Here's how the part is built. I have some questions about the finished solid (model axes, mm). Face numbers are marked on the shaded views. Round coordinates to 2 decimals unless told otherwise and drop trailing zeros. Loops run counter-clockwise (first coordinate to the right, second up) from the corner with the lowest first, then second, coordinate; pieces in that order, holes last. Notation, with made-up numbers: M -20,-7.5 L 5,-7.5 A9 ccw 5,-3.5 Z; hole C 31.5,84 d8. An arc over 180 degrees is marked long. One line per question, with ' | ' between items. Start each with the question number.
Autodesk Inventor part; units mm, degrees
ref_plane "YZ Plane" through (0, 0, 0) normal (1, 0, 0) x (0, 1, 0)
ref_plane "XZ Plane" through (0, 0, 0) normal (0, 1, 0) x (-1, 0, 0)
ref_plane "XY Plane" through (0, 0, 0) normal (0, 0, 1) x (1, 0, 0)
sketch "Skizze1" plane through (0, 0, 0) normal (0, 0, 1) x (1, 0, 0)
  line L0 (0, 0) -> (32, 0)
  line L1 (32, 0) -> (32, 59)
  line L2 (32, 59) -> (0, 59)
  line L3 (0, 59) -> (0, 0)
  dimension "d0" = 32
  dimension "d1" = 59
extrude "Extrusion1" add sketch "Skizze1" against normal blind 2
sketch "Skizze2" plane through (0, 0, -2) normal (0, 0, -1) x (-1, 0, 0)
  line L0 (-2.1, 2.1) -> (-29.9, 2.1)
  line L1 (-29.9, 2.1) -> (-29.9, 56.9)
  line L2 (-29.9, 56.9) -> (-2.1, 56.9)
  line L3 (-2.1, 56.9) -> (-2.1, 2.1)
  line L4 (0, 0) -> (0, 59) construction
  line L5 (-32, 0) -> (0, 0) construction
  point P0 (-2.1, 29.5)
  point P1 (0, 29.5)
  point P2 (-16, 2.1)
  point P3 (-16, 0)
  dimension "d4" = 2.1
  dimension "d5" = 2.1
extrude "Extrusion2" add sketch "Skizze2" along normal blind 2
sketch "Skizze3" plane through (0, 0, -4) normal (0, 0, -1) x (-1, 0, 0)
  circle A0 centre (-19.7, 39.4) radius 2.7
  line L0 (-32, 0) -> (0, 0)
  line L1 (-2.1, 2.1) -> (-2.1, 56.9)
  line L2 (-29.9, 56.9) -> (-29.9, 2.1)
  circle A1 centre (-19.7, 47.02) radius 2.7
  dimension "d8" = 5.4
  dimension "d9" = 39.4
  dimension "d11" = 10.2
  dimension "d12" = 5.4
  dimension "d13" = 7.62
extrude "Extrusion3" cut sketch "Skizze3" against normal through all
fillet "Rundung1" radius 1 4 edges at (16, 56.9, -4) (29.9, 29.5, -4) (2.1, 29.5, -4) (16, 2.1, -4)
fillet "Rundung2" radius 2 4 edges at (0, 59, -1) (0, 0, -1) (32, 59, -1) (32, 0, -1)
sketch "Skizze4" plane through (0, 0, -4) normal (0, 0, -1) x (-1, 0, 0)
  line L0 (-26, 31.9) -> (-6, 31.9)
  line L1 (-6, 31.9) -> (-6, 35.4)
  line L2 (-6, 35.4) -> (-26, 35.4)
  line L3 (-26, 35.4) -> (-26, 31.9)
  line L4 (-29.9, 2.1) -> (-2.1, 2.1)
  point P0 (0, 0)
  point P1 (-16, 31.9)
  point P2 (-16, 2.1)
  dimension "d18" = 20
  dimension "d19" = 3.5
  dimension "d20" = 29.8
extrude "Extrusion4" add sketch "Skizze4" along normal blind 6.01
sketch "Skizze6" plane through (6, 31.9, -4) normal (0, -1, 0) x (1, 0, 0)
  line L0 (0, -6.01) -> (2.5, -6.01)
  line L1 (2.5, -6.01) -> (0, -2)
  line L2 (0, -2) -> (0, -6.01)
  line L3 (20, 0) -> (0, 0) construction
  line L4 (10, 0) -> (10, 6.9424) construction
  line L5 (20, -6.01) -> (17.5, -6.01)
  line L6 (17.5, -6.01) -> (20, -2)
  line L7 (20, -2) -> (20, -6.01)
  point P0 (-6, 4)
  dimension "d29" = 2
  dimension "d30" = 2.5
  dimension "d31" = 4.01
extrude "Extrusion5" cut sketch "Skizze6" against normal up to surface (3.5 mm away)
properties part number "top"
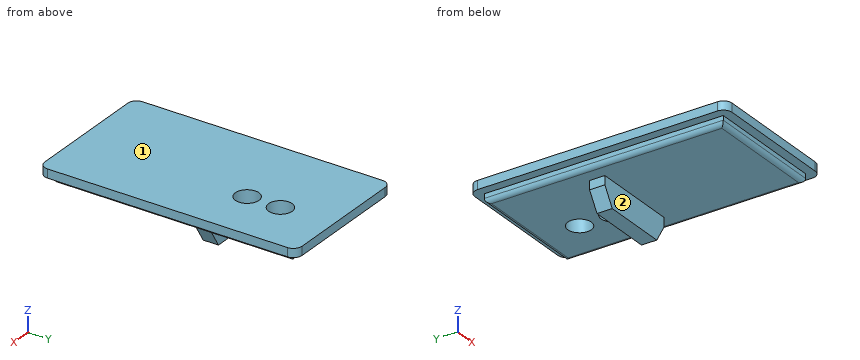
1) Imagine slicing it at B-B (x = 19.7). Write out the boundary of the cut face in (y, z).
2) Imagine slicing it at D-D (x = 11). Write out the boundary of the cut face in (y, z), then the cut area to 3 significant figures.
3) I'm going to push flat-ended pins straight in: pin 1 Ø2 at (x, z) = (18, -6) entering from +Y; pin 2 Ø6 at (y, z) = (49, -6) entering from -X; pin 3 Ø8.5 at (x, y) = (19.7, 39.4) entering from -Z; pin 4 Ø4 at (x, y) = (4.5, 29) entering from -Z. Where does each tip first touch, or does it pass through?
4) Please list where these lines run through material, in increasing order: L1, parallel to Y at x = 19.7, z = -0.9; L2, parallel to Y at x = 19.7, z = -2.15; L3, parallel to Z at x = 10, y = 25. Write a range as from..to.
5) Imagine slicing it at C-C (z = -0.75). Write out the boundary of the cut face in (x, y).
6) We'd pull the mould along Y, two halves only. Please class the marked faces 1 and 2: pulls with the +Y half, pulls with the -Y half, needs draft (parallel to the pull), parting line crosses it, or undercut.
7) Imagine slicing it at A-A (y = 39.4). Write out the boundary of the cut face in (x, z).
Results are:
1) outline: M 0,-2 L 2.1,-2 L 2.1,-3 A1 ccw 3.1,-4 L 31.9,-4 L 31.9,-10.01 L 35.4,-10.01 L 35.4,-4 L 36.7,-4 L 36.7,0 L 0,0 Z; M 42.1,-4 L 44.32,-4 L 44.32,0 L 42.1,0 Z; M 49.72,-4 L 55.9,-4 A1 ccw 56.9,-3 L 56.9,-2 L 59,-2 L 59,0 L 49.72,0 Z
2) outline: M 0,-2 L 2.1,-2 L 2.1,-3 A1 ccw 3.1,-4 L 31.9,-4 L 31.9,-10.01 L 35.4,-10.01 L 35.4,-4 L 55.9,-4 A1 ccw 56.9,-3 L 56.9,-2 L 59,-2 L 59,0 L 0,0 Z | area: 248 mm²
3) pin 1: y = 35.4 | pin 2: x = 2.1 | pin 3: z = -10.01 | pin 4: z = -4
4) L1: 0..36.7, 42.1..44.32, 49.72..59 | L2: 2.1..36.7, 42.1..44.32, 49.72..56.9 | L3: -4..0
5) outline: M 0,2 A2 ccw 2,0 L 30,0 A2 ccw 32,2 L 32,57 A2 ccw 30,59 L 2,59 A2 ccw 0,57 Z; hole C 19.7,39.4 d5.4; hole C 19.7,47.02 d5.4
6) face 1: needs draft | face 2: pulls with the -Y half
7) outline: M 0,-2 L 2.1,-2 L 2.1,-3 A1 ccw 3.1,-4 L 17,-4 L 17,0 L 0,0 Z; M 22.4,-4 L 28.9,-4 A1 ccw 29.9,-3 L 29.9,-2 L 32,-2 L 32,0 L 22.4,0 Z
